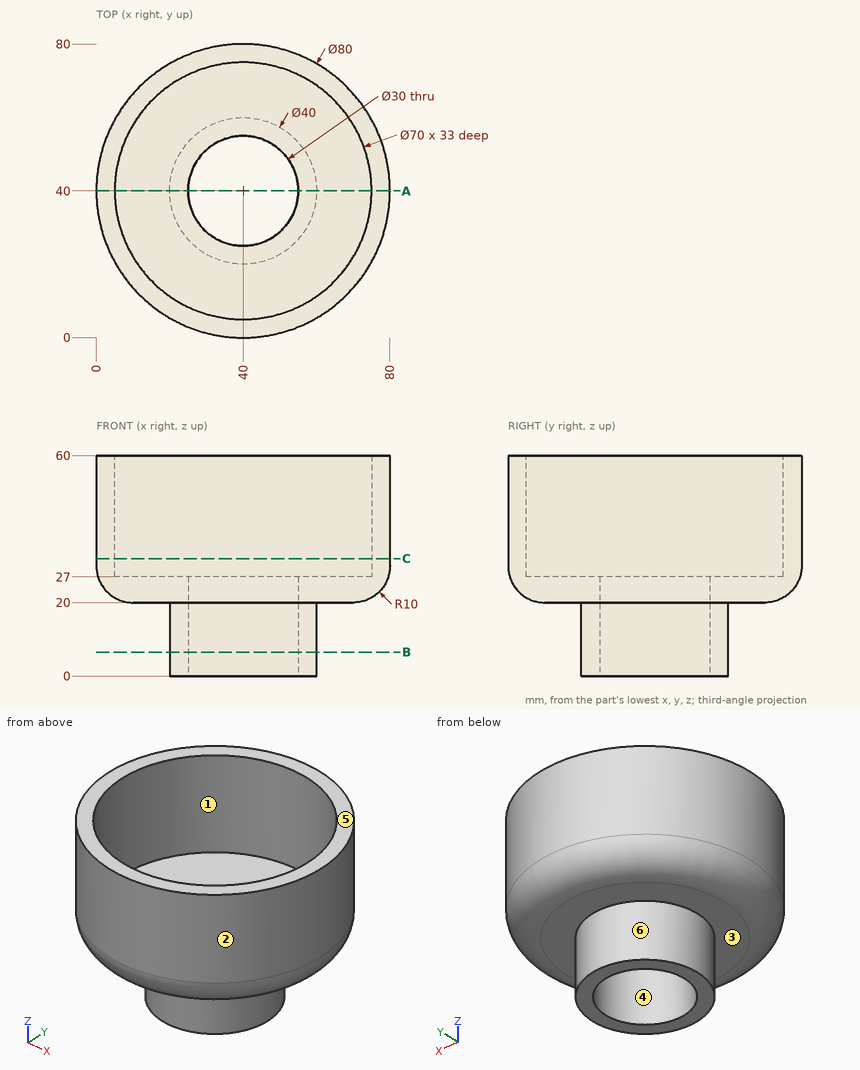
Print and shaded views of the part. All mm, measured from the part's lowest x, y and z. A direction names the side the tool comes from. Coordinates: 2 decimals unless noted, no trailing zeros. Loops run counter-clockwise (first coordinate to the right, second up) from the corner with the lowest first, then second, coordinate; pieces in that order, holes last. Notation, with made-up numbers: (55, 56) - (84, 56) arc R16 cw to (84, 81) - close; hole circle Ø8 at (21, 40). An arc over 180 degrees is marked (long way). Write item = value, one per line. Start each with the question number.
Item 1: Cut at A-A, the plane y = 40. Give the cut face in (x, z).
Item 2: Flat gauge pins, fed straight in: pin 1 Ø12 at (x, y) = (31.5, 36.5) entering from +Z; pin 2 Ø10 at (y, z) = (16.5, 50.5) entering from -X; pin 3 Ø3 at (x, z) = (28.5, 27) entering from +Y. Where does each tip first touch, or does it go through?
Item 3: Cut at B-B, the plane z = 6.5. Give the cut face in (x, y), and give its area (3 significant figures).
Item 4: Wall check: L1, parallel to X at y = 39, z = 39; L2, parallel to Y at x = 40, z = 16.5; L3, parallel to Y at x = 40, z = 52. Give the ranges that are in metal, low to high. Write a range as from..to.
Item 5: 3-axis set-ups, long thin cutter, end or side, ignore diameter. For the marked faces 1, 2 and 3: which of +Z, -Z, +X, -X, +Y, -Y reach the whole face in a straight line?
Item 6: Cut at C-C, the plane z = 32. Give the cut face in (x, y), and give its area (3 significant figures).
Item 7: Mould opens along Y. For the marked faces 4, 5 and 6 say: released by +Y, released by -Y, zero draft, split by the parting line, or undercut.
The answers:
q1.outline = (0, 30) arc R10 ccw to (10, 20) - (20, 20) - (20, 0) - (25, 0) - (25, 27) - (5, 27) - (5, 60) - (0, 60) - close; (55, 0) - (60, 0) - (60, 20) - (70, 20) arc R10 ccw to (80, 30) - (80, 60) - (75, 60) - (75, 27) - (55, 27) - close
q2.pin_1 = 27
q2.pin_2 = 4.54
q2.pin_3 = 78.42
q3.outline = circle Ø40 at (40, 40); hole circle Ø30 at (40, 40)
q3.area = 550 mm2
q4.L1 = 0.01..5.01, 74.99..79.99
q4.L2 = 20..25, 55..60
q4.L3 = 0..5, 75..80
q5.face_1 = +Z
q5.face_2 = +Z, -Z
q5.face_3 = -Z
q6.outline = circle Ø80 at (40, 40); hole circle Ø70 at (40, 40)
q6.area = 1,180 mm2
q7.face_4 = undercut
q7.face_5 = zero draft
q7.face_6 = split by the parting line
